Check sheet for the modelled part. Datum: model origin and axes. Units: mm. Face numbers are marked on the shaded views. A direction names the side the tool comes from. Round coordinates to 2 decimals unless told otherwise and drop trailing zeros. Order: outer loops, then holes, each group sorted by start corner. A loop starts at its lowest first (then second) coordinate and runs counter-clockwise, first axis right, second up. Notation, with made-up numbers: (63.25, 78) -> (89.25, 78) arc R26 ccw to (89.25, 92) -> close; hole circle Ø7 at (81, 0). An arc over 180 degrees is marked (long way). Answer in a Markdown table with one row per item. Add a question column.
1. Material ranges on L1, parallel to Z at x = 40.5, y = 194.5; L2, parallel to X at y = 205.5, z = 31.5; L3, parallel to X at y = 242, z = 13.5, recorded low to high. Write a range as from..to.
2. Sectioned sample at D-D, the plane z = 35. Count the separate pieces of the cut face and the enclosed holes in it, then the cut area to 3 significant figures.
3. Sectioned sample at B-B, the plane x = 55. Record the boundary of the cut face in (y, z).
4. Sectioned sample at C-C, the plane y = 197.5. Record the boundary of the cut face in (x, z).
5. Draft check along X on the marked faces 3, 4 and 5. Enter one of: +X half, -X half, draft (parallel to the pull), parting line (faces both ways), or undercut.
6. Access from +Z, -Z, +X, -X, +Y, -Y to the whole of each face (thin tool, end or side, straight path). Record for the marked faces 1 and 2.
7. Depth check by flat-ended pin: P1, Ø6, axis at x = 38, y = 233, coming from the +Z side; P2, Ø10, axis at x = 61, y = 234, coming from the +Z side; P3, Ø1.5, axis at x = 15.5, y = 243.5, coming from the +Z side; P4, Ø12, axis at x = 29, z = 49, coming from the -Y side. Enter the tip coordinate at first touch or a pass-through.
8. Sectioned sample at A-A, the plane z = 25.5. Record the boundary of the cut face in (x, y), then the cut area to 3 significant figures.
```python
from build123d import *

# Parameters (mm, degrees)
SKETCH024_W     = 95
SKETCH024_H     = 95
PAD016_DEPTH    = 5
PAD017_DEPTH    = 95
SKETCH029_R     = 30
POCKET009_DEPTH = 102.501
FILLET022_R     = 5
FILLET023_R     = 2


with BuildPart() as part:
    # Sketch024 → Pad016 (new body)
    with BuildSketch(Plane.XY):
        Rectangle(SKETCH024_W, SKETCH024_H)
    extrude(amount=PAD016_DEPTH)

    # Sketch025 (on DatumPlane) → Pad017 (join)
    with BuildSketch(Plane(origin=(0, 47.5, 0), x_dir=(-1, 0, 0), z_dir=(0, 1, 0))):
        Polygon((-47, 5), (-17, 56.961524), (-14, 56.961524), (-44, 5), align=None)
        Polygon((-24, 5), (6, 56.961524), (9, 56.961524), (-21, 5), align=None)
        Polygon((-1, 5), (29, 56.961524), (32, 56.961524), (2, 5), align=None)
        Polygon((22, 5), (52, 56.961524), (55, 56.961524), (25, 5), align=None)
    extrude(amount=-PAD017_DEPTH)

    # Sketch029 (on DatumPlane) → Pocket009 (cut, through all)
    with BuildSketch(Plane.YZ.offset(47.5)):
        with Locations((0, 60)):
            Circle(SKETCH029_R)
    extrude(amount=-POCKET009_DEPTH, mode=Mode.SUBTRACT)

    # Fillet022
    fillet022_edges = [part.edges().sort_by_distance(p)[0] for p in [
        (15.5, -47.5, 56.961524),
        (15.5, -29.845731, 56.961524),
        (-7.5, -47.5, 56.961524),
        (-7.5, -29.845731, 56.961524),
        (-30.5, -47.5, 56.961524),
        (-30.5, -29.845731, 56.961524),
        (-53.5, -47.5, 56.961524),
        (-53.5, -29.845731, 56.961524),
        (15.5, 29.845731, 56.961524),
        (15.5, 47.5, 56.961524),
        (-7.5, 29.845731, 56.961524),
        (-7.5, 47.5, 56.961524),
        (-30.5, 29.845731, 56.961524),
        (-30.5, 47.5, 56.961524),
        (-53.5, 29.845731, 56.961524),
        (-53.5, 47.5, 56.961524),
    ]]
    fillet(fillet022_edges, radius=FILLET022_R)

    # Fillet023
    fillet023_edges = [part.edges().sort_by_distance(p)[0] for p in [
        (0, -47.5, 0),
        (47.5, 0, 0),
        (0, 47.5, 0),
        (-47.5, 0, 0),
    ]]
    fillet(fillet023_edges, radius=FILLET023_R)


with BuildPart() as part_1:
    # Body011 placement: moved
    add(part.part.moved(Location((48, 233, 0))))


solid = part_1.part
```
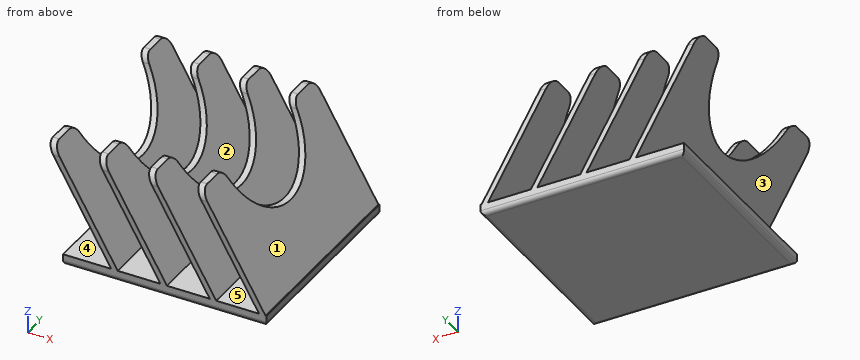
Answer key:
| question | item | result |
|---|---|---|
| 1 | L1 | z = 0..5, 14.53..19.72, 54.36..56.96 |
| 1 | L2 | x = 7.7..10.7, 30.7..33.7, 53.7..56.7, 76.7..79.7 |
| 1 | L3 | x = 18.09..21.09, 41.09..44.09, 64.09..67.09, 87.09..90.09 |
| 2 | separate pieces | 8 |
| 2 | enclosed holes | 0 |
| 2 | area | 742 mm² |
| 3 | outline | (185.5, 2) arc R2 ccw to (187.5, 0) -> (278.5, 0) arc R2 ccw to (280.5, 2) -> (280.5, 5) -> (185.5, 5) -> close; (185.5, 29.25) -> (280.5, 29.25) -> (280.5, 34.44) -> (248.71, 34.44) arc R30 cw to (217.29, 34.44) -> (185.5, 34.44) -> close |
| 4 | outline | (-7, 56.96) -> (23, 5) -> (0.5, 5) -> (0.5, 2) arc R2 ccw to (2.5, 0) -> (93.5, 0) arc R2 ccw to (95.5, 2) -> (95.5, 5) -> (95, 5) -> (65, 56.96) -> (62, 56.96) -> (92, 5) -> (72, 5) -> (42, 56.96) -> (39, 56.96) -> (69, 5) -> (49, 5) -> (19, 56.96) -> (16, 56.96) -> (46, 5) -> (26, 5) -> (-4, 56.96) -> close |
| 5 | face 3 | -X half |
| 5 | face 4 | draft |
| 5 | face 5 | undercut |
| 6 | face 1 | +Z, +X, +Y, -Y |
| 6 | face 2 | +Y, -Y |
| 7 | P1 | stops at z = 29.25 |
| 7 | P2 | stops at z = 30.33 |
| 7 | P3 | stops at z = 24.49 |
| 7 | P4 | stops at y = 185.5 |
| 8 | outline | (11.16, 185.5) -> (14.16, 185.5) -> (14.16, 280.5) -> (11.16, 280.5) -> close; (34.16, 185.5) -> (37.16, 185.5) -> (37.16, 280.5) -> (34.16, 280.5) -> close; (57.16, 185.5) -> (60.16, 185.5) -> (60.16, 280.5) -> (57.16, 280.5) -> close; (80.16, 185.5) -> (83.16, 185.5) -> (83.16, 280.5) -> (80.16, 280.5) -> close |
| 8 | area | 1,140 mm² |
